```python
from build123d import *

# Parameters (mm, degrees)
SKT_BASE_W_MOUNTING_HOLES_R           = 1.85
EXT_BASE_PLATE_W_MOUNTING_HOLES_DEPTH = 5
SKT_UPWARD_RIDGE_W                    = 86.25
SKT_UPWARD_RIDGE_H                    = 5
EXT_UPWARD_FLANGE_DEPTH               = 65
EXT_PIX_PLATFORM_DEPTH                = 5
PIX_MOUNT_HOLES_REACH                 = 91.702
SKETCH7_R                             = 1.625
SKETCH8_W                             = 40
SKETCH8_H                             = 5
GPS_FLANGE_DEPTH                      = 55
SKETCH9_R                             = 1.3
GPS_PLATFORM_DEPTH                    = 5
BRACING_DEPTH                         = 5


with BuildPart() as part:
    # Skt - Base w mounting holes → Ext - Base Plate w Mounting Holes (new body)
    with BuildSketch(Plane(origin=(0, 0, 0), x_dir=(1, 0, 0), z_dir=(0, 1, 0))):
        with BuildLine():
            Line((-38.125, 23.7), (38.125, 23.7))
            ThreePointArc((38.125, 23.7), (41.660533906, 22.235533906), (43.125, 18.7))
            Line((43.125, 18.7), (43.125, -18.7))
            ThreePointArc((43.125, -18.7), (41.660533906, -22.235533906), (38.125, -23.7))
            Line((38.125, -23.7), (-38.125, -23.7))
            ThreePointArc((-38.125, -23.7), (-41.660533906, -22.235533906), (-43.125, -18.7))
            Line((-43.125, -18.7), (-43.125, 18.7))
            ThreePointArc((-43.125, 18.7), (-41.660533906, 22.235533906), (-38.125, 23.7))
        make_face()
        with Locations(Location((-38.125, 18.7, 0), (0, 0, 270))):
            Circle(SKT_BASE_W_MOUNTING_HOLES_R, mode=Mode.SUBTRACT)
        with Locations(Location((38.125, 18.7, 0), (0, 0, 270))):
            Circle(SKT_BASE_W_MOUNTING_HOLES_R, mode=Mode.SUBTRACT)
        with Locations(Location((38.125, -18.7, 0), (0, 0, 270))):
            Circle(SKT_BASE_W_MOUNTING_HOLES_R, mode=Mode.SUBTRACT)
        with Locations(Location((-38.125, -18.7, 0), (0, 0, 270))):
            Circle(SKT_BASE_W_MOUNTING_HOLES_R, mode=Mode.SUBTRACT)
    extrude(amount=EXT_BASE_PLATE_W_MOUNTING_HOLES_DEPTH)

    # Skt - Upward Ridge → Ext - Upward Flange (add)
    with BuildSketch(Plane(origin=(0, 5, 0), x_dir=(1, 0, 0), z_dir=(0, 1, 0))):
        Rectangle(SKT_UPWARD_RIDGE_W, SKT_UPWARD_RIDGE_H)
    extrude(amount=EXT_UPWARD_FLANGE_DEPTH)

    # Skt - GPS Nest → Ext - PIX Platform (add)
    with BuildSketch(Plane(origin=(0, 70, 0), x_dir=(1, 0, 0), z_dir=(0, 1, 0))):
        with BuildLine():
            Line((1.875, 23.5), (38.125, 23.5))
            ThreePointArc((38.125, 23.5), (41.660533906, 22.035533906), (43.125, 18.5))
            Line((43.125, 18.5), (43.125, -18.5))
            ThreePointArc((43.125, -18.5), (41.660533906, -22.035533906), (38.125, -23.5))
            Line((38.125, -23.5), (1.875, -23.5))
            ThreePointArc((1.875, -23.5), (-1.660533906, -22.035533906), (-3.125, -18.5))
            Line((-3.125, -18.5), (-3.125, 18.5))
            ThreePointArc((-3.125, 18.5), (-1.660533906, 22.035533906), (1.875, 23.5))
        make_face()
    extrude(amount=EXT_PIX_PLATFORM_DEPTH)

    # Sketch7 → Pix Mount Holes (cut, up to next)
    with BuildSketch(Plane(origin=(0, 75, 0), x_dir=(1, 0, 0), z_dir=(0, 1, 0)), mode=Mode.PRIVATE) as pix_mount_holes_sk1:
        with Locations(Location((7.975, 15.25, 0), (0, 0, 270))):
            Circle(SKETCH7_R)
    pix_mount_holes_tool1 = extrude(pix_mount_holes_sk1.sketch, amount=-PIX_MOUNT_HOLES_REACH, mode=Mode.PRIVATE) & part.part
    # Sketch7 → Pix Mount Holes (cut, up to next)
    with BuildSketch(Plane(origin=(0, 75, 0), x_dir=(1, 0, 0), z_dir=(0, 1, 0)), mode=Mode.PRIVATE) as pix_mount_holes_sk2:
        with Locations(Location((38.125, 15.25, 0), (0, 0, 270))):
            Circle(SKETCH7_R)
    pix_mount_holes_tool2 = extrude(pix_mount_holes_sk2.sketch, amount=-PIX_MOUNT_HOLES_REACH, mode=Mode.PRIVATE) & part.part
    # Sketch7 → Pix Mount Holes (cut, up to next)
    with BuildSketch(Plane(origin=(0, 75, 0), x_dir=(1, 0, 0), z_dir=(0, 1, 0)), mode=Mode.PRIVATE) as pix_mount_holes_sk3:
        with Locations(Location((38.125, -15.25, 0), (0, 0, 270))):
            Circle(SKETCH7_R)
    pix_mount_holes_tool3 = extrude(pix_mount_holes_sk3.sketch, amount=-PIX_MOUNT_HOLES_REACH, mode=Mode.PRIVATE) & part.part
    # Sketch7 → Pix Mount Holes (cut, up to next)
    with BuildSketch(Plane(origin=(0, 75, 0), x_dir=(1, 0, 0), z_dir=(0, 1, 0)), mode=Mode.PRIVATE) as pix_mount_holes_sk4:
        with Locations(Location((7.975, -15.25, 0), (0, 0, 270))):
            Circle(SKETCH7_R)
    pix_mount_holes_tool4 = extrude(pix_mount_holes_sk4.sketch, amount=-PIX_MOUNT_HOLES_REACH, mode=Mode.PRIVATE) & part.part
    add(pix_mount_holes_tool1.solids().sort_by_distance((7.975, 75, -15.25))[0], mode=Mode.SUBTRACT)
    add(pix_mount_holes_tool2.solids().sort_by_distance((38.125, 75, -15.25))[0], mode=Mode.SUBTRACT)
    add(pix_mount_holes_tool3.solids().sort_by_distance((38.125, 75, 15.25))[0], mode=Mode.SUBTRACT)
    add(pix_mount_holes_tool4.solids().sort_by_distance((7.975, 75, 15.25))[0], mode=Mode.SUBTRACT)

    # Sketch8 → GPS Flange (add)
    with BuildSketch(Plane(origin=(0, 70, 0), x_dir=(1, 0, 0), z_dir=(0, 1, 0))):
        with Locations((-23.125, 0)):
            Rectangle(SKETCH8_W, SKETCH8_H)
    extrude(amount=GPS_FLANGE_DEPTH)

    # Sketch9 → GPS Platform (add)
    with BuildSketch(Plane(origin=(0, 125, 0), x_dir=(1, 0, 0), z_dir=(0, 1, 0))):
        with BuildLine():
            Line((-38.125, 23.7), (-8.125, 23.7))
            ThreePointArc((-8.125, 23.7), (-4.589466094, 22.235533906), (-3.125, 18.7))
            Line((-3.125, 18.7), (-3.125, -18.7))
            ThreePointArc((-3.125, -18.7), (-4.589466094, -22.235533906), (-8.125, -23.7))
            Line((-8.125, -23.7), (-38.125, -23.7))
            ThreePointArc((-38.125, -23.7), (-41.660533906, -22.235533906), (-43.125, -18.7))
            Line((-43.125, -18.7), (-43.125, 18.7))
            ThreePointArc((-43.125, 18.7), (-41.660533906, 22.235533906), (-38.125, 23.7))
        make_face()
        with Locations(Location((-39.125, 16.5, 0), (0, 0, 270))):
            Circle(SKETCH9_R, mode=Mode.SUBTRACT)
        with Locations(Location((-7.125, 16.5, 0), (0, 0, 270))):
            Circle(SKETCH9_R, mode=Mode.SUBTRACT)
        with Locations(Location((-7.125, -16.5, 0), (0, 0, 270))):
            Circle(SKETCH9_R, mode=Mode.SUBTRACT)
        with Locations(Location((-39.125, -16.5, 0), (0, 0, 270))):
            Circle(SKETCH9_R, mode=Mode.SUBTRACT)
    extrude(amount=GPS_PLATFORM_DEPTH)

    # Sketch10 → Bracing (add)
    with BuildSketch(Plane.ZY.offset(43.125)):
        Polygon((-2.5, 5), (-2.5, 125), (-12.5, 125), (-14.5, 5), align=None)
        Polygon((2.5, 125), (2.5, 5), (14.5, 5), (12.5, 125), align=None)
    extrude(amount=-BRACING_DEPTH)


solid = part.part
```
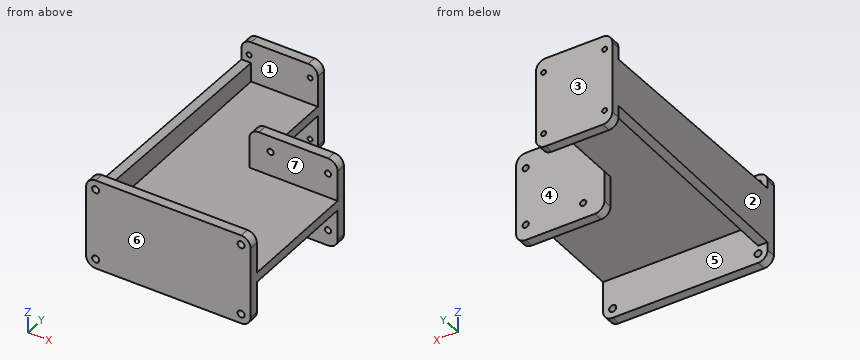
Source: CAD feature listing. Evaluate the final solid. Frame: model axes, mm. Face numbers are marked on the shaded views. A direction names the side the tool comes from. Round coordinates to 2 decimals unless told otherwise and drop trailing zeros. Loops run counter-clockwise (first coordinate to the right, second up) from the corner with the lowest first, then second, coordinate; pieces in that order, holes last.
(1) Contact query for flat-ended pins moving along their axis: pin 1 Ø5 at (x, y) = (16.5, 55) entering from +Z; pin 2 Ø12 at (y, z) = (42.5, -16.5) entering from -X (3 decimals); pin 3 Ø12 at (x, z) = (3, 14.5) entering from +Y; pin 4 Ø6 at (y, z) = (86, -9.5) entering from +X (3 decimals). Output: stop coordinate, or through.
From the geometry:
pin 1: stops at z = 2.5
pin 2: stops at x = -43.125
pin 3: stops at y = 75
pin 4: stops at x = -38.125
(2) Section query D-D (x = -23.5). Output: boundary loops of the cut face in (y, z), and give its area (3 significant figures).
From the geometry:
outline: (0, -23.7) - (5, -23.7) - (5, -2.5) - (125, -2.5) - (125, -23.7) - (130, -23.7) - (130, 23.7) - (125, 23.7) - (125, 2.5) - (5, 2.5) - (5, 23.7) - (0, 23.7) - close
area: 1,070 mm2
(3) Pull-direction query (Y, two-part tool) for the marked faces 1, 2 and 3; classes: +Y half, -Y half, draft (parallel to the pull), parting line (faces both ways), or undercut.
From the geometry:
face 1: undercut
face 2: draft
face 3: +Y half
(4) Section query A-A (z = -4). Output: boundary loops of the cut face in (x, y) (3 decimals).
From the geometry:
outline: (-43.125, 0) - (43.125, 0) - (43.125, 5) - (-38.125, 5) - (-38.125, 125) - (-3.125, 125) - (-3.125, 130) - (-43.125, 130) - close; (-3.125, 70) - (43.125, 70) - (43.125, 75) - (-3.125, 75) - close
(5) Section query C-C (y = 44). Output: boundary loops of the cut face in (x, z) (3 decimals).
From the geometry:
outline: (-43.125, -13.85) - (-38.125, -13.85) - (-38.125, -2.5) - (43.125, -2.5) - (43.125, 2.5) - (-38.125, 2.5) - (-38.125, 13.85) - (-43.125, 13.85) - close
(6) Section query B-B (x = 20). Output: boundary loops of the cut face in (y, z), and give its area (3 significant figures).
From the geometry:
outline: (0, -23.7) - (5, -23.7) - (5, -2.5) - (70, -2.5) - (70, -23.5) - (75, -23.5) - (75, 23.5) - (70, 23.5) - (70, 2.5) - (5, 2.5) - (5, 23.7) - (0, 23.7) - close
area: 797 mm2
(7) Material intervals for probe 1 along X at (y, z) = (73, -15) (3 decimals); probe 2 along X at (y, z) = (126.25, 16.5) (3 decimals); probe 3 along Y at (x, z) = (-24, 7.5), sorted ascending.
From the geometry:
probe 1: x = -3.125 to 6.369, 9.581 to 36.519, 39.731 to 43.125
probe 2: x = -43.125 to -40.425, -37.825 to -8.425, -5.825 to -3.125
probe 3: y = 0 to 5, 125 to 130
(8) Access query for the marked faces 4, 5, 6 and 7. Directions: +Z, -Z, +X, -X, +Y, -Y. A direction counts if a zero-diameter tool reaches every point of the face in a straight line with its end or side. Return the directions, or none.
From the geometry:
face 4: +Z, -Z, +X, +Y
face 5: -Z, +X
face 6: +Z, -Z, +X, -X, -Y
face 7: +Z, +X
